from build123d import *

# Parameters (mm, degrees)
SKETCH1_W            = 498.348
SKETCH1_H            = 165.1
BOSS_EXTRUDE1_DEPTH  = 1.5875
BOSS_EXTRUDE2_DEPTH  = 3.175
CUT_EXTRUDE1_DEPTH   = 4.175
LPATTERN1_COUNT      = 5
LPATTERN1_PITCH      = 88.9
CUT_EXTRUDE2_START   = -4.175
CUT_EXTRUDE2_DEPTH   = 5.175
LPATTERN2_COUNT      = 2
LPATTERN2_PITCH      = 38.1
SKETCH5_W            = 3.175
SKETCH5_H            = 88.9
CUT_EXTRUDE3_DEPTH   = 4.175
SKETCH6_W            = 2.286
SKETCH6_H            = 107.442
CUT_EXTRUDE4_DEPTH   = 4.175
LPATTERN3_COUNT      = 4
LPATTERN3_PITCH      = 98.8568
SKETCH8_W            = 50.8
SKETCH8_H            = 3.175
BOSS_EXTRUDE3_DEPTH  = 3.175
SKETCH9_R            = 11.05
CUT_EXTRUDE5_DEPTH   = 4.175
M6_CLEARANCE_HOLE1_D = 6.6
LPATTERN4_COUNT      = 3
LPATTERN4_PITCH      = 98.8568
LPATTERN4_COL_COUNT  = 3
LPATTERN4_COL_PITCH  = 98.8568
M3_CLEARANCE_HOLE1_D = 3.4
M4_CLEARANCE_HOLE1_D = 4.5
CUT_EXTRUDE6_DEPTH   = 4.175


with BuildPart() as part:
    # Sketch1 → Boss-Extrude1 (new body, symmetric)
    with BuildSketch(Plane(origin=(0, 0, 0), x_dir=(0, 0, -1), z_dir=(1, 0, 0))):
        Rectangle(SKETCH1_W, SKETCH1_H)
    extrude(amount=BOSS_EXTRUDE1_DEPTH, both=True)

    # Sketch2 → Boss-Extrude2 (add)
    with BuildSketch(Plane(origin=(1.5875, 0, 0), x_dir=(0, 0, -1), z_dir=(1, 0, 0))):
        Polygon((192.024, -139.7), (249.174, -82.55), (-249.174, -82.55), (-249.174, -139.7), align=None)
    extrude(amount=-BOSS_EXTRUDE2_DEPTH)

    # Sketch3 → Cut-Extrude1 (cut, through all)
    with BuildSketch(Plane.ZY.offset(1.5875)):
        with BuildLine():
            ThreePointArc((222.877, -130.81), (216.603382579, -128.211382579), (219.202, -134.485))
            Line((219.202, -134.485), (219.202, -130.81))
            Line((219.202, -130.81), (222.877, -130.81))
        make_face()
        with BuildLine():
            Line((219.202, -130.81), (219.202, -134.485))
            ThreePointArc((219.202, -134.485), (221.800617421, -133.408617421), (222.877, -130.81))
            Line((222.877, -130.81), (219.202, -130.81))
        make_face()
    cut_extrude1 = extrude(amount=-CUT_EXTRUDE1_DEPTH, mode=Mode.SUBTRACT)

    # LPattern1: Cut-Extrude1 ×5
    with Locations(*[(0, 0, -i * LPATTERN1_PITCH) for i in range(1, LPATTERN1_COUNT)]):
        add(cut_extrude1, mode=Mode.SUBTRACT)

    # Sketch4 → Cut-Extrude2 (cut)
    with BuildSketch(Plane.ZY.offset(1.5875).offset(CUT_EXTRUDE2_START)):
        with BuildLine():
            ThreePointArc((-194.635179285, -117.249359697), (-199.716540899, -113.854102415), (-200.908796706, -119.847977118))
            Line((-200.908796706, -119.847977118), (-198.310179285, -117.249359697))
            Line((-198.310179285, -117.249359697), (-195.711561864, -119.847977118))
            ThreePointArc((-195.711561864, -119.847977118), (-194.914922003, -118.655721311), (-194.635179285, -117.249359697))
        make_face()
        with BuildLine():
            Line((-198.310179285, -117.249359697), (-200.908796706, -119.847977118))
            ThreePointArc((-200.908796706, -119.847977118), (-198.310179285, -120.924359697), (-195.711561864, -119.847977118))
            Line((-195.711561864, -119.847977118), (-198.310179285, -117.249359697))
        make_face()
    cut_extrude2 = extrude(amount=CUT_EXTRUDE2_DEPTH, mode=Mode.SUBTRACT)

    # LPattern2: Cut-Extrude2 ×2
    with Locations(*[Vector(0, 0.707106781, -0.707106781) * (i * LPATTERN2_PITCH) for i in range(1, LPATTERN2_COUNT)]):
        add(cut_extrude2, mode=Mode.SUBTRACT)

    # Sketch5 → Cut-Extrude3 (cut, through all)
    with BuildSketch(Plane(origin=(1.5875, 0, 0), x_dir=(0, 0, -1), z_dir=(1, 0, 0))):
        with Locations((247.5865, 38.1)):
            Rectangle(SKETCH5_W, SKETCH5_H)
        with Locations((-247.5865, 38.1)):
            Rectangle(SKETCH5_W, SKETCH5_H)
    extrude(amount=-CUT_EXTRUDE3_DEPTH, mode=Mode.SUBTRACT)

    # Sketch6 → Cut-Extrude4 (cut, through all)
    with BuildSketch(Plane(origin=(1.5875, 0, 0), x_dir=(0, 0, -1), z_dir=(1, 0, 0))):
        with Locations((148.2852, 28.829)):
            Rectangle(SKETCH6_W, SKETCH6_H)
    cut_extrude4 = extrude(amount=-CUT_EXTRUDE4_DEPTH, mode=Mode.SUBTRACT)

    # LPattern3: Cut-Extrude4 ×4
    with Locations(*[(0, 0, i * LPATTERN3_PITCH) for i in range(1, LPATTERN3_COUNT)]):
        add(cut_extrude4, mode=Mode.SUBTRACT)

    # Sketch8 → Boss-Extrude3 (add)
    with BuildSketch(Plane(origin=(1.5875, 0, 0), x_dir=(0, 0, -1), z_dir=(1, 0, 0))):
        with Locations((0, 84.1375)):
            Rectangle(SKETCH8_W, SKETCH8_H)
    extrude(amount=-BOSS_EXTRUDE3_DEPTH)

    # Sketch9 → Cut-Extrude5 (cut, through all)
    with BuildSketch(Plane(origin=(1.5875, 0, 0), x_dir=(0, 0, -1), z_dir=(1, 0, 0))):
        with Locations((-42.9768, -96.7994)):
            Circle(SKETCH9_R)
    extrude(amount=-CUT_EXTRUDE5_DEPTH, mode=Mode.SUBTRACT)

    # M6 Clearance Hole1 (through all)
    with Locations(Plane(origin=(1.5875, 0, 0), x_dir=(0, 0, -1), z_dir=(1, 0, 0))):
        with Locations((0, -73.8124)):
            m6_clearance_hole1 = Hole(M6_CLEARANCE_HOLE1_D / 2)

    # LPattern4: M6 Clearance Hole1 ×3
    with Locations(*[(0, 0, i * LPATTERN4_PITCH) for i in range(1, LPATTERN4_COUNT)]):
        add(m6_clearance_hole1, mode=Mode.SUBTRACT)

    # LPattern4 col: M6 Clearance Hole1 ×3
    with Locations(*[(0, 0, -i * LPATTERN4_COL_PITCH) for i in range(1, LPATTERN4_COL_COUNT)]):
        add(m6_clearance_hole1, mode=Mode.SUBTRACT)

    # M3 Clearance Hole1 (through all)
    with Locations(Plane(origin=(1.5875, 0, 0), x_dir=(0, 0, -1), z_dir=(1, 0, 0))):
        with Locations((11.674, -77.315), (11.674, -103.315), (57.674, -103.315), (57.674, -77.315)):
            Hole(M3_CLEARANCE_HOLE1_D / 2)

    # M4 Clearance Hole1 (through all)
    with Locations(Plane(origin=(1.5875, 0, 0), x_dir=(0, 0, -1), z_dir=(1, 0, 0))):
        with Locations((-25.0163, -78.8389), (-60.9373, -78.8389), (-60.9373, -114.7599), (-25.0163, -114.7599)):
            Hole(M4_CLEARANCE_HOLE1_D / 2)

    # Sketch14 → Cut-Extrude6 (cut, through all)
    with BuildSketch(Plane(origin=(1.5875, 0, 0), x_dir=(0, 0, -1), z_dir=(1, 0, 0))):
        with BuildLine():
            Line((45.674, -101.565), (23.674, -101.565))
            ThreePointArc((23.674, -101.565), (12.424, -90.315), (23.674, -79.065))
            Line((23.674, -79.065), (45.674, -79.065))
            ThreePointArc((45.674, -79.065), (56.924, -90.315), (45.674, -101.565))
        make_face()
    extrude(amount=-CUT_EXTRUDE6_DEPTH, mode=Mode.SUBTRACT)


solid = part.part
Can you work these out from the model? Positions are in its coordinate system, mm. A direction names the side the tool comes from. Give positions to 0.01 mm unless a question says otherwise; leave off trailing zeros. Order: outer loops, then holes, each group sorted by start corner. A loop starts at its lowest first (then second) coordinate and runs counter-clockwise, first axis right, second up. Notation, with made-up numbers: M 8,80.25 L 54,80.25 A7 cw 54,93.25 Z; hole C 51,33 d2. An arc over 180 degrees is marked long. Use a Markdown table: item, result. Add a question column.
Item 1: Suppose I cut it at B-B (x = 0.8). Count the separate pieces of the cut face and the enclosed holes in it, then the cut area to 3 significant figures.
Item 2: For faces 1 (the cylindrical face through (0.022, -90.562, -12.427)), 2 (the flat face through (-1.588, -25, 3)), which set-ups out of +Z, -Z, +X, -X, +Y, -Y let a thin tool reach every point of the face, with its end or its side?
Item 3: Will these pins go through, and if not, where does the flat tip stop? pin 1 (4 mm diameter, centred on y = -73.81, z = 0, fed in from -X); pin 2 (1 mm diameter, centred on x = 0.5, y = 20, fed in from -Z); pin 3 (1.6 mm diameter, centred on x = 0.5, z = -40, fed in from +Y); pin 4 (1.5 mm diameter, centred on x = 1, y = -101, fed in from -Z).
Item 4: If I drill on L1, parallel to Z at x = -0.3, y = -130.81; L2, parallel to Z at x = -1.05, y = 8; L3, parallel to Y at x = -0.6, z = 130, over which ranges is the centre line in solid material (lowest first)? Write a range as [from, to].
Item 5: We'd pull the mould along Y, two halves only. Please class faces 3 (the cylindrical face through (0.02, -90.07, -56.92)), 4 (the flat face through (1.588, -25, 3)), 5 (the flat face through (0.022, -111.525, -220.199)): +Y half, -Y half, draft (parallel to the pull), parting line (faces both ways), or undercut.
Item 6: Suppose I cut it at A-A (y = 36). List the corners of the cut face in (x, z) for me.
Answer sheet:
| question | item | result |
|---|---|---|
| 1 | separate pieces | 1 |
| 1 | enclosed holes | 22 |
| 1 | area | 106,000 mm² |
| 2 | face 1 | +X, -X |
| 2 | face 2 | +Z, -Z, -X, +Y, -Y |
| 3 | pin 1 | passes through |
| 3 | pin 2 | stops at z = -246 |
| 3 | pin 3 | stops at y = 82.55 |
| 3 | pin 4 | stops at z = -231.47 |
| 4 | L1 | z = [-200.91, -140.07], [-132.72, -51.17], [-43.82, 37.73], [45.08, 126.63], [133.98, 215.53], [222.88, 249.17] |
| 4 | L2 | z = [-246, -149.43], [-147.14, -50.57], [-48.29, 48.29], [50.57, 147.14], [149.43, 246] |
| 4 | L3 | y = [-139.7, -134.47], [-127.15, 82.55] |
| 5 | face 3 | undercut |
| 5 | face 4 | draft |
| 5 | face 5 | -Y half |
| 6 | outline | M -1.59,-246 L 1.59,-246 L 1.59,-149.43 L -1.59,-149.43 Z; M -1.59,-147.14 L 1.59,-147.14 L 1.59,-50.57 L -1.59,-50.57 Z; M -1.59,-48.29 L 1.59,-48.29 L 1.59,48.29 L -1.59,48.29 Z; M -1.59,50.57 L 1.59,50.57 L 1.59,147.14 L -1.59,147.14 Z; M -1.59,149.43 L 1.59,149.43 L 1.59,246 L -1.59,246 Z |
